```python
from build123d import *

# Parameters (mm, degrees)
SKETCH1_R           = 34
SKETCH1_R_2         = 1.5
SKETCH1_R_3         = 3.5
SKETCH1_W           = 14
SKETCH1_H           = 14
BOSS_EXTRUDE1_DEPTH = 2


with BuildPart() as part:
    # Sketch1 → Boss-Extrude1 (new body)
    with BuildSketch(Plane.XY):
        Circle(SKETCH1_R)
        with Locations((30, 0)):
            Circle(SKETCH1_R_2, mode=Mode.SUBTRACT)
        with Locations((-7.5, -12.990381057)):
            Circle(SKETCH1_R_2, mode=Mode.SUBTRACT)
        with Locations((-7.5, 12.990381057)):
            Circle(SKETCH1_R_2, mode=Mode.SUBTRACT)
        with Locations((-17.5, 20)):
            Circle(SKETCH1_R_3, mode=Mode.SUBTRACT)
        with Locations(Location((17.5, 20, 0), (0, 0, 180))):
            Circle(SKETCH1_R_3, mode=Mode.SUBTRACT)
        with Locations(Location((-17.5, -20, 0), (0, 0, 180))):
            Circle(SKETCH1_R_3, mode=Mode.SUBTRACT)
        with Locations((17.5, -20)):
            Circle(SKETCH1_R_3, mode=Mode.SUBTRACT)
        with Locations((20.845079102, 9.72022002)):
            Circle(SKETCH1_R_3, mode=Mode.SUBTRACT)
        with Locations((0, -23)):
            Circle(SKETCH1_R_3, mode=Mode.SUBTRACT)
        with Locations((-20.845079102, 9.72022002)):
            Circle(SKETCH1_R_3, mode=Mode.SUBTRACT)
        Rectangle(SKETCH1_W, SKETCH1_H, mode=Mode.SUBTRACT)
    extrude(amount=BOSS_EXTRUDE1_DEPTH)


solid = part.part
```
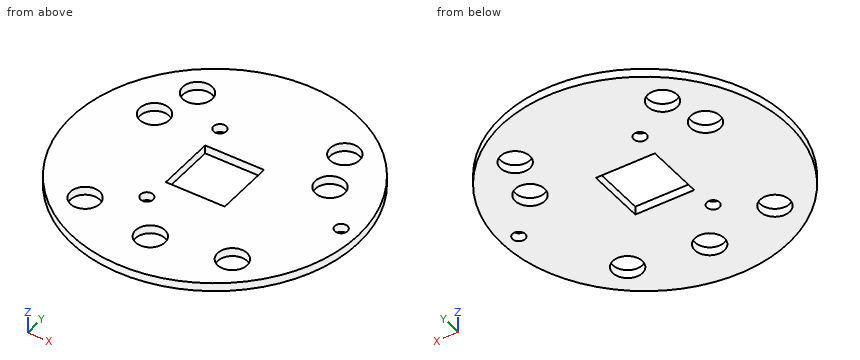
Check sheet for the modelled part. Datum: model origin and axes. Units: mm. Round coordinates to 2 decimals unless told otherwise and drop trailing zeros. Loops run counter-clockwise (first coordinate to the right, second up) from the corner with the lowest first, then second, coordinate; pieces in that order, holes last. Notation, with made-up numbers: (82.25, -37) -> (100.25, -37) arc R18 ccw to (100.25, -32) -> close; hole circle Ø7 at (-4.5, 63). An arc over 180 degrees is marked (long way). Answer in a Markdown table with one row per item.
Q1. Sectioned sample at C-C on z = 1.05. Give the number of separate pieces and of enclosed holes in the cut face, then the cut area to 3 significant figures.
Data:
| item | result |
|---|---|
| separate pieces | 1 |
| enclosed holes | 11 |
| area | 3,150 mm^2 |
Q2. Thickness scan on L1, parallel to Y at x = 0, z = 1.2; L2, parallel to Y at x = 3, z = 0.15; L3, parallel to X at y = -18, z = 1.1. Record the ranges inside material, lowest first.
Data:
| item | result |
|---|---|
| L1 | y = -34 to -26.5, -19.5 to -7, 7 to 34 |
| L2 | y = -33.87 to -24.8, -21.2 to -7, 7 to 33.87 |
| L3 | x = -28.84 to -20.37, -14.63 to 14.63, 20.37 to 28.84 |
Q3. Sectioned sample at A-A on x = 0. Enter the section's corners in (y, z).
Data:
| item | result |
|---|---|
| outline | (-34, 0) -> (-26.5, 0) -> (-26.5, 2) -> (-34, 2) -> close; (-19.5, 0) -> (-7, 0) -> (-7, 2) -> (-19.5, 2) -> close; (7, 0) -> (34, 0) -> (34, 2) -> (7, 2) -> close |
Q4. Sectioned sample at D-D on y = -25. Enter the section's corners in (x, z), then the cut area to 3 significant figures.
Data:
| item | result |
|---|---|
| outline | (-23.04, 0) -> (-2.87, 0) -> (-2.87, 2) -> (-23.04, 2) -> close; (2.87, 0) -> (23.04, 0) -> (23.04, 2) -> (2.87, 2) -> close |
| area | 80.7 mm^2 |
Q5. Sectioned sample at B-B on y = 0. Enter the section's corners in (x, z).
Data:
| item | result |
|---|---|
| outline | (-34, 0) -> (-7, 0) -> (-7, 2) -> (-34, 2) -> close; (7, 0) -> (28.5, 0) -> (28.5, 2) -> (7, 2) -> close; (31.5, 0) -> (34, 0) -> (34, 2) -> (31.5, 2) -> close |
Q6. Go/stop test with flat-tipped pins: P1, Ø1, axis at y = 1, z = 0.5, coming from the -X side; P2, Ø1, axis at y = 6, z = 1, coming from the +X side. Record where each tip stops, or that it passes through.
Data:
| item | result |
|---|---|
| P1 | stops at x = -34 |
| P2 | stops at x = 33.55 |
